Answer from the drawing. Dimensions are ordinates in mm from the lowest x, y and z of the part. Coordinates: 2 decimals unless noted, no trailing zeros. Order: outer loops, then holes, each group sorted by start corner. A loop starts at its lowest first (then second) coordinate and runs counter-clockwise, first axis right, second up. Notation, with made-up numbers: M 77,-5 L 88,-5 A17 cw 88,5 Z; hole C 78,-12 d7. An arc over 180 degrees is marked long. One line per question, with ' | ' between items. Start each with the question number.
1) Find section A-A, the plane x = 22.86. Write down the section's boundary in (y, z), plus the area to 3 significant figures.
2) Consider probe 1 along Z at (x, y) = (27.94, 0.85); probe 2 along X at (y, z) = (0.5, 2.54); probe 3 along X at (y, z) = (0.5, 1.75). Determine where each line is inside the solid, lowest interval first.
3) Find section B-B, the plane z = 15. Write down the section's boundary in (x, y), plus the area to 3 significant figures.
4) Given P1, Ø0.5, axis at y = 1, z = 8.5, coming from the +X side (3 decimals), flat-ended and moving along its own axis, determine where the tip first touches the part or whether it passes through.
5) Find section D-D, the plane x = 18. Write down the section's boundary in (y, z), plus the area to 3 significant figures.
6) Find section C-C, the plane y = 0.75. Count the separate pieces of the cut face and the enclosed holes in it, plus the area to 3 significant figures.
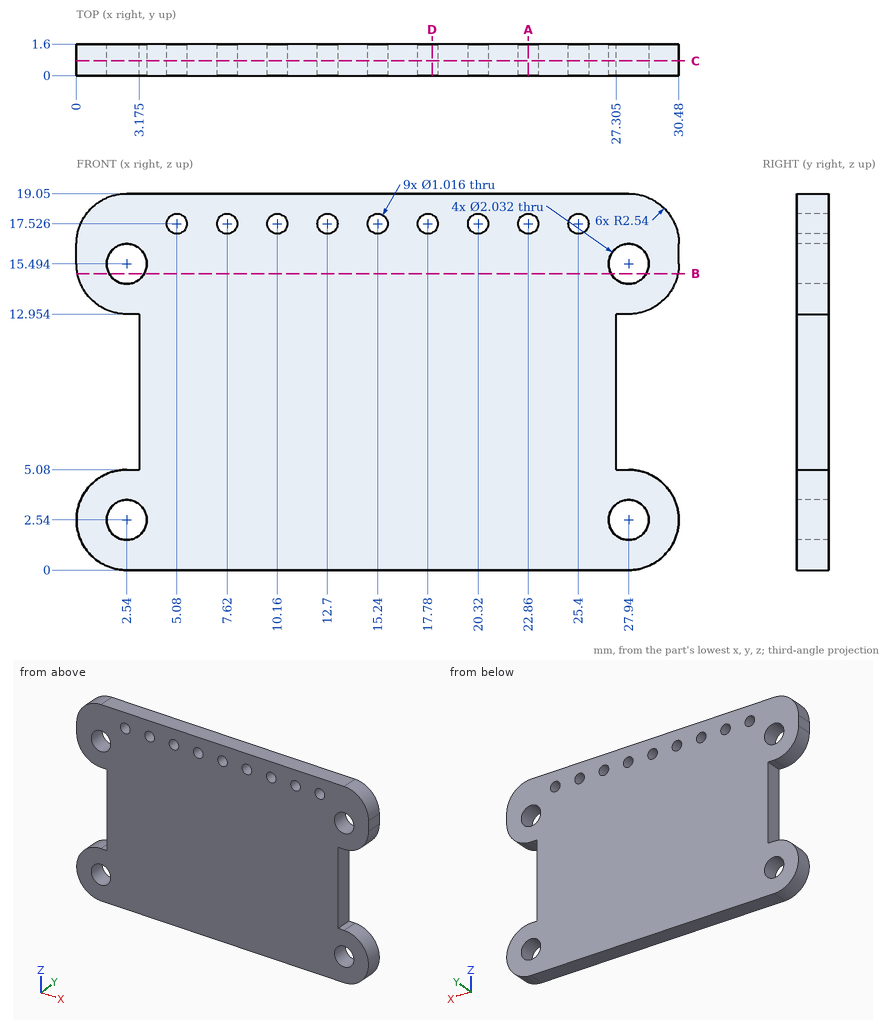
Report:
1) outline: M 0,0 L 1.6,0 L 1.6,17.02 L 0,17.02 Z; M 0,18.03 L 1.6,18.03 L 1.6,19.05 L 0,19.05 Z | area: 28.9 mm^2
2) probe 1: z = 0 to 1.52, 3.56 to 5.08, 12.95 to 14.48, 16.51 to 19.05 | probe 2: x = 0 to 1.52, 3.56 to 26.92, 28.96 to 30.48 | probe 3: x = 0.13 to 1.9, 3.18 to 27.3, 28.58 to 30.35
3) outline: M 0.05,0 L 1.65,0 L 1.65,1.6 L 0.05,1.6 Z; M 3.43,0 L 27.05,0 L 27.05,1.6 L 3.43,1.6 Z; M 28.83,0 L 30.43,0 L 30.43,1.6 L 28.83,1.6 Z | area: 42.9 mm^2
4) P1: stops at x = 27.305
5) outline: M 0,0 L 1.6,0 L 1.6,17.07 L 0,17.07 Z; M 0,17.98 L 1.6,17.98 L 1.6,19.05 L 0,19.05 Z | area: 29.0 mm^2
6) separate pieces: 1 | enclosed holes: 13 | area: 499 mm^2
